from build123d import *

# Parameters (mm, degrees)
F0_W        = 17.78
F0_H        = 37.338
F1_DEPTH    = 1.27
F2_R        = 1.143
F3_DEPTH    = 1.27
F5_DEPTH    = 25.4
F6_T1_DEPTH = 1.27
F6_T3_DEPTH = 5.715
F6_T5_DEPTH = 5.715
F6_T7_DEPTH = 5.715
F6_T9_DEPTH = 5.2860926284
F8_DEPTH    = 5.334
F9_R        = 0.381
F10_DEPTH   = 1.27
F11_R       = 0.381
F12_DEPTH   = 1.27
F14_DEPTH   = 4.953
F15_R       = 0.254
F16_W       = 3.429
F16_H       = 2.8956
F17_DEPTH   = 1.27
F18_R       = 0.8509
F19_DEPTH   = 0.4064


# Not quite as in the source:
# - a fillet or chamfer that OpenCascade refuses, or shapes differently, is made with other operations: its cross-section is extruded or revolved along the edge and cut away or added


with BuildPart() as f1:
    # F0 (on Top) → F1 (new body)
    with BuildSketch(Plane.XY):
        Rectangle(F0_W, F0_H)
    extrude(amount=F1_DEPTH)

    # F2 (on face) → F3 (cut, through all)
    with BuildSketch(Plane.XY.offset(1.27)):
        with Locations((6.985, 16.891)):
            Circle(F2_R)
        with Locations((-6.985, 16.891)):
            Circle(F2_R)
        with Locations((0, -9.017)):
            Circle(F2_R)
    extrude(amount=-F3_DEPTH, mode=Mode.SUBTRACT)

    # F4 (on face) → F5 (cut)
    with BuildSketch(Plane.XY.offset(1.27)):
        Polygon((-8.89, -17.78), (-8.89, -18.669), (-7.493, -18.669), (-8.382, -17.78), align=None)
        Polygon((8.89, -18.669), (8.89, -17.78), (4.699, -17.78), (3.81, -18.669), align=None)
    extrude(amount=-F5_DEPTH, mode=Mode.SUBTRACT)

    # F6: fillet of radius 0.889 on 5 edges, made by hand

    # F6_s2 → F6_t1 (join)
    with BuildSketch(Plane.XY):
        with BuildLine():
            ThreePointArc((5.0672358569, -17.78), (4.7270302856, -17.8476710956), (4.4386179285, -18.0403820715))
            Line((4.4386179285, -18.0403820715), (4.699, -17.78))
            Line((4.699, -17.78), (5.0672358569, -17.78))
        make_face()
    extrude(amount=F6_T1_DEPTH)

    # F6_s4 → F6_t3 (cut)
    with BuildSketch(Plane.XY.offset(-2.2225)):
        with BuildLine():
            ThreePointArc((8.001, 18.669), (8.6296179285, 18.4086179285), (8.89, 17.78))
            Line((8.89, 17.78), (8.89, 18.669))
            Line((8.89, 18.669), (8.001, 18.669))
        make_face()
    extrude(amount=F6_T3_DEPTH, mode=Mode.SUBTRACT)

    # F6_s6 → F6_t5 (cut)
    with BuildSketch(Plane.XY.offset(-2.2225)):
        with BuildLine():
            ThreePointArc((-8.001, 18.669), (-8.6296179285, 18.4086179285), (-8.89, 17.78))
            Line((-8.89, 17.78), (-8.89, 18.669))
            Line((-8.89, 18.669), (-8.001, 18.669))
        make_face()
    extrude(amount=F6_T5_DEPTH, mode=Mode.SUBTRACT)

    # F6_s8 → F6_t7 (cut)
    with BuildSketch(Plane.XY.offset(-2.2225)):
        with BuildLine():
            ThreePointArc((8.001, -17.78), (8.6296179285, -17.5196179285), (8.89, -16.891))
            Line((8.89, -16.891), (8.89, -17.78))
            Line((8.89, -17.78), (8.001, -17.78))
        make_face()
    extrude(amount=F6_T7_DEPTH, mode=Mode.SUBTRACT)

    # F6_s10 → F6_t9 (cut)
    with BuildSketch(Plane.XY.offset(-2.0080463142)):
        with BuildLine():
            ThreePointArc((-8.382, -17.78), (-8.7523421325, -17.4519719624), (-8.89, -16.9767814743))
            Line((-8.89, -16.9767814743), (-8.89, -17.78))
            Line((-8.89, -17.78), (-8.382, -17.78))
        make_face()
    extrude(amount=F6_T9_DEPTH, mode=Mode.SUBTRACT)

    # F7 (on face) → F8 (join)
    with BuildSketch(Plane(origin=(0, 18.669, 0), x_dir=(-1, 0, 0), z_dir=(0, 1, 0))):
        with BuildLine():
            Line((3.81, 3.9624), (0, 3.9624))
            Line((0, 3.9624), (-3.81, 3.9624))
            Line((-3.81, 3.9624), (-3.81, 2.54))
            ThreePointArc((-3.81, 2.54), (-3.4380256121, 1.6419743879), (-2.54, 1.27))
            Line((-2.54, 1.27), (0, 1.27))
            Line((0, 1.27), (2.54, 1.27))
            ThreePointArc((2.54, 1.27), (3.4380256121, 1.6419743879), (3.81, 2.54))
            Line((3.81, 2.54), (3.81, 3.9624))
        make_face()
    extrude(amount=-F8_DEPTH)

    # F9 (on face) → F10 (cut, through all)
    with BuildSketch(Plane.XY.offset(1.27)):
        with Locations((7.62, 14.351)):
            Circle(F9_R)
        with Locations((7.62, 11.811)):
            Circle(F9_R)
        with Locations((7.62, 9.271)):
            Circle(F9_R)
        with Locations((7.62, 6.731)):
            Circle(F9_R)
        with Locations((7.62, 4.191)):
            Circle(F9_R)
        with Locations((7.62, 1.651)):
            Circle(F9_R)
        with Locations((7.62, -0.889)):
            Circle(F9_R)
        with Locations((7.62, -3.429)):
            Circle(F9_R)
        with Locations((7.62, -5.969)):
            Circle(F9_R)
        with Locations((7.62, -8.509)):
            Circle(F9_R)
        with Locations((7.62, -11.049)):
            Circle(F9_R)
        with Locations((7.62, -13.589)):
            Circle(F9_R)
        with Locations((-7.62, -13.589)):
            Circle(F9_R)
        with Locations((-7.62, -11.049)):
            Circle(F9_R)
        with Locations((-7.62, -8.509)):
            Circle(F9_R)
        with Locations((-7.62, -5.969)):
            Circle(F9_R)
        with Locations((-7.62, -3.429)):
            Circle(F9_R)
        with Locations((-7.62, -0.889)):
            Circle(F9_R)
        with Locations((-7.62, 1.651)):
            Circle(F9_R)
        with Locations((-7.62, 4.191)):
            Circle(F9_R)
        with Locations((-7.62, 6.731)):
            Circle(F9_R)
        with Locations((-7.62, 9.271)):
            Circle(F9_R)
        with Locations((-7.62, 11.811)):
            Circle(F9_R)
        with Locations((-7.62, 14.351)):
            Circle(F9_R)
    extrude(amount=-F10_DEPTH, mode=Mode.SUBTRACT)

    # F11 (on face) → F12 (cut, through all)
    with BuildSketch(Plane.XY.offset(1.27)):
        with Locations((-6.35, -16.383)):
            Circle(F11_R)
        with Locations((-3.81, -16.383)):
            Circle(F11_R)
        with Locations((-1.27, -16.383)):
            Circle(F11_R)
        with Locations((1.27, -16.383)):
            Circle(F11_R)
        with Locations((3.81, -16.383)):
            Circle(F11_R)
        with Locations((6.35, -16.383)):
            Circle(F11_R)
    extrude(amount=-F12_DEPTH, mode=Mode.SUBTRACT)

    # F13 (on face) → F14 (cut, through all)
    with BuildSketch(Plane(origin=(0, 18.669, 0), x_dir=(-1, 0, 0), z_dir=(0, 1, 0))):
        with BuildLine():
            Line((-2.54, 1.6509998994), (2.54, 1.6509998994))
            ThreePointArc((2.54, 1.6509998994), (3.1686179996, 1.9113820004), (3.4290001006, 2.54))
            Line((3.4290001006, 2.54), (3.4290001006, 3.5814001006))
            Line((3.4290001006, 3.5814001006), (-3.4290001006, 3.5814001006))
            Line((-3.4290001006, 3.5814001006), (-3.4290001006, 2.54))
            ThreePointArc((-3.4290001006, 2.54), (-3.1686179996, 1.9113820004), (-2.54, 1.6509998994))
        make_face()
    extrude(amount=-F14_DEPTH, mode=Mode.SUBTRACT)

    # F15
    f15_edges = [f1.edges().sort_by_distance(p)[0] for p in [
        (3.81, 16.002, 3.9624),
        (-3.81, 16.002, 3.9624),
    ]]
    fillet(f15_edges, radius=F15_R)

    # F16 (on face) → F17 (join)
    with BuildSketch(Plane.XY.offset(1.27)):
        with Locations((0, -12.2682)):
            Rectangle(F16_W, F16_H)
    extrude(amount=F17_DEPTH)

    # F18 (on face) → F19 (join)
    with BuildSketch(Plane.XY.offset(2.54)):
        with Locations((0, -12.2682)):
            Circle(F18_R)
    extrude(amount=F19_DEPTH)


solid = f1.part
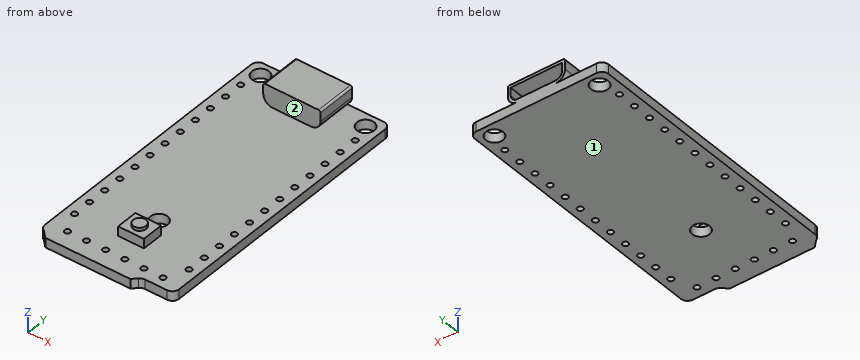
Part model, mm, in its own coordinate system. Face numbers are marked on the shaded views. Coordinates: 2 decimals unless noted, no trailing zeros. Loops run counter-clockwise (first coordinate to the right, second up) from the corner with the lowest first, then second, coordinate; pieces in that order, holes last. Notation, with made-up numbers: (88, 89) -> (136, 89) arc R31 cw to (136, 116) -> close; hole circle Ø6 at (1.25, -9.75). An arc over 180 degrees is marked (long way). Use a Markdown table: item, result. Add a question column.
Item 1: Band-saw the part on C-C on y = -4.5. Write the cut outline in (x, z), plus the area to 3 significant figures.
Item 2: Pull direction Y, two halves, no side cores. Call the marked faces 1 and 2: +Y half, -Y half, draft (parallel to the pull), parting line (faces both ways), or undercut.
Item 3: Probe probe 1 along X at (y, z) = (1.5, 1.2); probe 2 along X at (y, z) = (11.5, 0.5); probe 3 along Y at (x, z) = (1, 3) (3 decimals). List the from-to ranges inside material, lowest first.
Item 4: Flat gauge pins, fed straight in: P1, Ø3, axis at x = -5.5, y = -9.5, coming from the +Z side; P2, Ø0.9, axis at y = 17, z = 3, coming from the +X side; P3, Ø1.4, axis at x = -6.985, y = 16.891, coming from the +Z side; P4, Ø1, axis at y = -12, z = 2, coming from the +X side. Where does each tip first touch, or does it go through?
Item 5: Band-saw the part on B-B on x = 6.35. Write the cut outline in (y, z).
Item 6: Band-saw the part on A-A on x = 0. Write the cut outline in (y, z) (3 decimals), plus the area to 3 significant figures.
Item 7: Band-saw the part on D-D on z = 0.7. Give the number of separate pieces and of enclosed holes in the cut face, plus the area to 3 significant figures.
Geometry says:
| question | item | result |
|---|---|---|
| 1 | outline | (-8.89, 0) -> (8.89, 0) -> (8.89, 1.27) -> (-8.89, 1.27) -> close |
| 1 | area | 22.6 mm² |
| 2 | face 1 | draft |
| 2 | face 2 | undercut |
| 3 | probe 1 | -8.89 to -7.97, -7.27 to 7.27, 7.97 to 8.89 |
| 3 | probe 2 | -8.89 to -7.84, -7.4 to 7.4, 7.84 to 8.89 |
| 3 | probe 3 | 13.335 to 13.716 |
| 4 | P1 | z = 1.27 |
| 4 | P2 | x = 3.81 |
| 4 | P3 | through |
| 4 | P4 | x = 1.71 |
| 5 | outline | (-17.78, 0) -> (-16.76, 0) -> (-16.76, 1.27) -> (-17.78, 1.27) -> close; (-16, 0) -> (15.94, 0) -> (15.94, 1.27) -> (-16, 1.27) -> close; (17.84, 0) -> (18.67, 0) -> (18.67, 1.27) -> (17.84, 1.27) -> close |
| 6 | outline | (-18.669, 0) -> (-10.16, 0) -> (-10.16, 1.27) -> (-10.82, 1.27) -> (-10.82, 2.54) -> (-11.417, 2.54) -> (-11.417, 2.946) -> (-13.119, 2.946) -> (-13.119, 2.54) -> (-13.716, 2.54) -> (-13.716, 1.27) -> (-18.669, 1.27) -> close; (-7.874, 0) -> (18.669, 0) -> (18.669, 1.651) -> (13.716, 1.651) -> (13.716, 3.581) -> (18.669, 3.581) -> (18.669, 3.962) -> (13.335, 3.962) -> (13.335, 1.27) -> (-7.874, 1.27) -> close |
| 6 | area | 53.7 mm² |
| 7 | separate pieces | 1 |
| 7 | enclosed holes | 33 |
| 7 | area | 632 mm² |
